Here's how the part is built. I have some questions about the finished solid (model axes, mm). Give positions to 0.01 mm unless a question says otherwise; leave off trailing zeros. Loops run counter-clockwise (first coordinate to the right, second up) from the corner with the lowest first, then second, coordinate; pieces in that order, holes last.
Q1. If we section it at B-B (x = 94): Please give me the cut outline in (y, z).
Q2. Will these pins go through, and if not, where does the flat tip stop? P1, Ø2, axis at y = -2.5, z = 119, coming from the -X side; P2, Ø4, axis at x = -53, y = -2.5, coming from the -Z side; P3, Ø6, axis at x = 46, z = 79, coming from the -Y side; P4, Ø3.5, axis at y = 1.5, z = 43.5, coming from the -X side.
Q3. I need wall thicknesses on line 1 (X direction, y = 0.5, z = 9); line 2 (Y direction, x = -16, z = 63.5); line 3 (Z direction, x = -5, y = -0.5). Which ranges of each line are inside material? Lowest first, please.
Q4. If we section it at A-A (z = 13): Please give me the cut outline in (x, y), plus the area to 3 significant figures.
from build123d import *

# Parameters (mm, degrees)
BOSS_EXTRUDE1_DEPTH = 3.2
SKETCH3_R           = 12.3
BOSS_EXTRUDE2_DEPTH = 3.2
SKETCH4_R           = 4
BOSS_EXTRUDE3_DEPTH = 4


with BuildPart() as part:
    # Sketch1 → Boss-Extrude1 (new body)
    with BuildSketch(Plane(origin=(0, 0, 0), x_dir=(1, 0, 0), z_dir=(0, 1, 0))):
        Polygon((-71.199297972, 0), (119.800702028, 0), (119.800702028, -90), (46.272924854, -150.155348756), (-15.035731115, -153.181069815), (-74.399297972, -109), (-74.399297972, -65), (-71.199297972, -65), align=None)
    extrude(amount=BOSS_EXTRUDE1_DEPTH)

    # Sketch3 → Boss-Extrude2 (add)
    with BuildSketch(Plane.XZ):
        with Locations(Location((-5.399297972, 108.199281837, 0), (0, 0, 270))):
            Circle(SKETCH3_R)
    extrude(amount=BOSS_EXTRUDE2_DEPTH)

    # Sketch4 → Boss-Extrude3 (add)
    with BuildSketch(Plane.XZ.offset(3.2)):
        with Locations(Location((-5.399297972, 108.199281837, 0), (0, 0, 270))):
            Circle(SKETCH4_R)
    extrude(amount=BOSS_EXTRUDE3_DEPTH)


solid = part.part
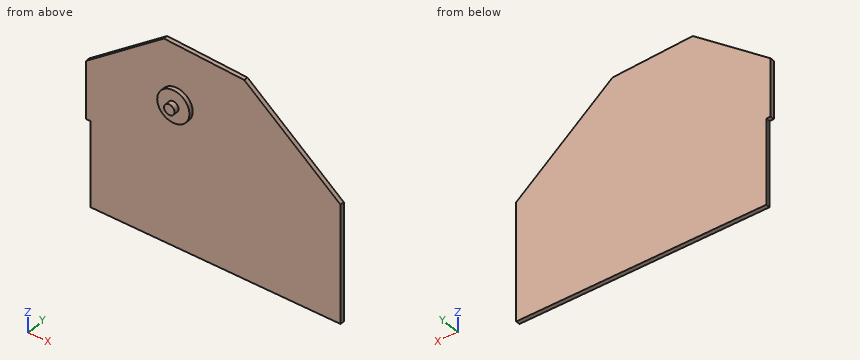
Check sheet entries:
1. outline: (0, 0) - (3.2, 0) - (3.2, 111.11) - (0, 111.11) - close
2. P1: stops at x = -12.83
2. P2: passes through
2. P3: stops at y = 0
2. P4: stops at x = -71.2
3. line 1: x = -71.2 to 119.8
3. line 2: y = 0 to 3.2
3. line 3: z = 95.91 to 120.49
4. outline: (-71.2, 0) - (119.8, 0) - (119.8, 3.2) - (-71.2, 3.2) - close
4. area: 611 mm2
